Verification items for this drawing (mm, ordinates from the low corner). Round coordinates to 2 decimals unless told otherwise and drop trailing zeros. Loops run counter-clockwise (first coordinate to the right, second up) from the corner with the lowest first, then second, coordinate; pieces in that order, holes last. Notation, with made-up numbers: M -31,-26.5 L -18,-26.5 A24 ccw -18,0.5 Z; hole C 77,0 d4. An arc over 180 degrees is marked long. One line per item, written item: value.
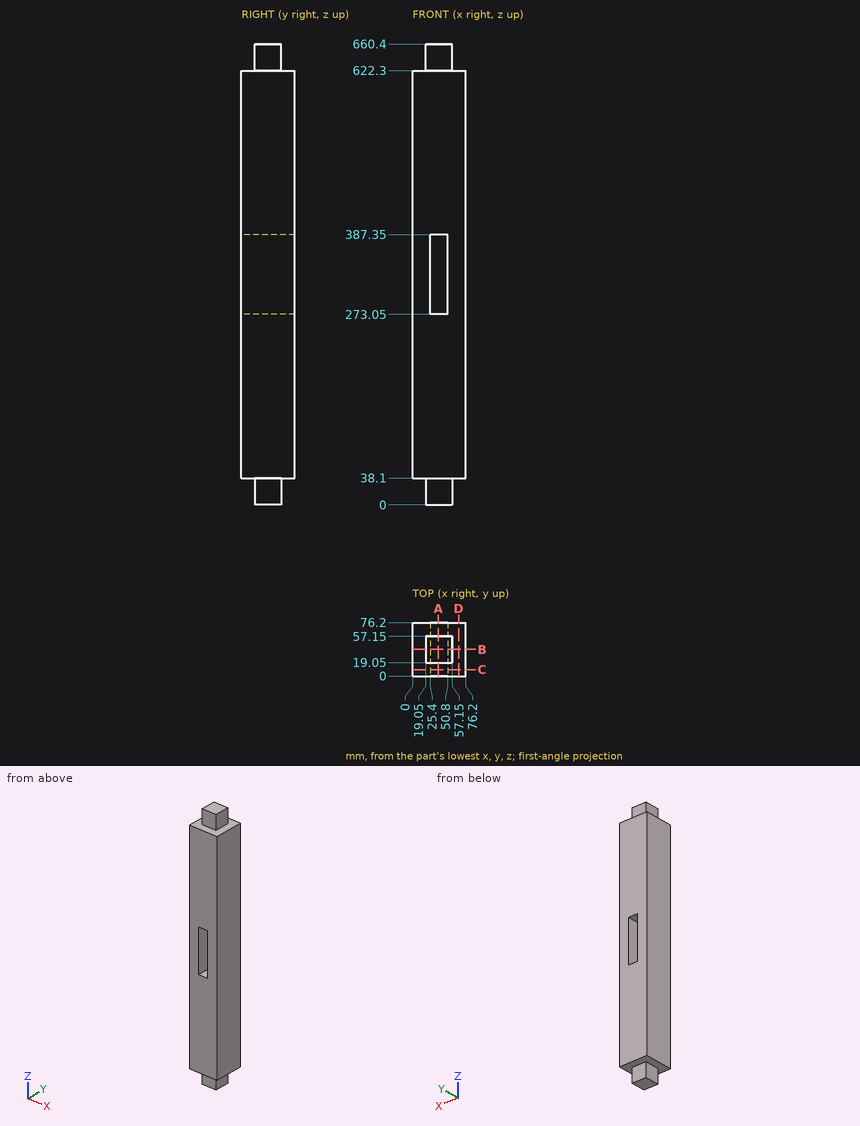
(1) Thickness scan on L1, parallel to X at y = 50, z = 333; L2, parallel to Z at x = 33, y = 43.5; L3, parallel to Z at x = 39, y = 59.5. Record the ranges inside material, lowest first. Write a range as from..to.
Completed:
L1: x = 0..25.4, 50.8..76.2
L2: z = 0..273.05, 387.35..660.4
L3: z = 38.1..273.05, 387.35..622.3
(2) Sectioned sample at D-D on x = 66. Enter the section's corners in (y, z), and give its area (3 significant figures).
Completed:
outline: M 0,38.1 L 76.2,38.1 L 76.2,622.3 L 0,622.3 Z
area: 44,500 mm^2
(3) Depth check by flat-ended pin: pin 1 Ø11.5 at (y, z) = (41, 17) entering from +X; pin 2 Ø11.5 at (x, z) = (37, 9.5) entering from -Y; pin 3 Ø2 at (x, y) = (63, 49) entering from -Z. Enter the tip coordinate at first touch or a pass-through.
Completed:
pin 1: stops at x = 57.15
pin 2: stops at y = 19.05
pin 3: stops at z = 38.1
(4) Sectioned sample at C-C on y = 9. Enter the section's corners in (x, z), and give its area (3 significant figures).
Completed:
outline: M 0,38.1 L 76.2,38.1 L 76.2,622.3 L 0,622.3 Z; hole M 25.4,273.05 L 50.8,273.05 L 50.8,387.35 L 25.4,387.35 Z
area: 41,600 mm^2
(5) Sectioned sample at B-B on y = 38. Enter the section's corners in (x, z), and give its area (3 significant figures).
Completed:
outline: M 0,38.1 L 19.05,38.1 L 19.05,0 L 57.15,0 L 57.15,38.1 L 76.2,38.1 L 76.2,622.3 L 57.15,622.3 L 57.15,660.4 L 19.05,660.4 L 19.05,622.3 L 0,622.3 Z; hole M 25.4,273.05 L 50.8,273.05 L 50.8,387.35 L 25.4,387.35 Z
area: 44,500 mm^2
(6) Sectioned sample at A-A on x = 37. Enter the section's corners in (y, z), and give its area (3 significant figures).
Completed:
outline: M 0,38.1 L 19.05,38.1 L 19.05,0 L 57.15,0 L 57.15,38.1 L 76.2,38.1 L 76.2,273.05 L 0,273.05 Z; M 0,387.35 L 76.2,387.35 L 76.2,622.3 L 57.15,622.3 L 57.15,660.4 L 19.05,660.4 L 19.05,622.3 L 0,622.3 Z
area: 38,700 mm^2
